Geometry: final body of the model. Coordinates: model frame, mm. A direction names the side the tool comes from. Give positions to 0.01 mm unless a question says otherwise; leave off trailing zeros. Loops run counter-clockwise (first coordinate to the right, second up) from the corner with the lowest first, then second, coordinate; pieces in that order, holes last. Notation, with made-up numbers: M -4.75,-9.75 L 12.25,-9.75 A13 ccw 12.25,7.25 Z; hole C 2.5,36.25 d3. An arc over 180 degrees is marked long. Put each result on its own line as item: value.
```python
from build123d import *

# Parameters (mm, degrees)
SKETCH2_W           = 42
SKETCH2_H           = 13.8
BOSS_EXTRUDE1_DEPTH = 2
SKETCH3_W           = 2
SKETCH3_H           = 13.8
BOSS_EXTRUDE2_DEPTH = 10
BOSS_EXTRUDE3_DEPTH = 2
SKETCH5_R           = 2.5
CUT_EXTRUDE1_DEPTH  = 2
SKETCH6_R           = 1.25
CUT_EXTRUDE2_DEPTH  = 2


with BuildPart() as part:
    # Sketch2 → Boss-Extrude1 (new body)
    with BuildSketch(Plane(origin=(0, 0, 0), x_dir=(1, 0, 0), z_dir=(0, 1, 0))):
        Rectangle(SKETCH2_W, SKETCH2_H)
    extrude(amount=BOSS_EXTRUDE1_DEPTH)

    # Sketch3 → Boss-Extrude2 (add)
    with BuildSketch(Plane.XZ):
        with Locations((-20, 0)):
            Rectangle(SKETCH3_W, SKETCH3_H)
        with Locations((20, 0)):
            Rectangle(SKETCH3_W, SKETCH3_H)
    extrude(amount=BOSS_EXTRUDE2_DEPTH)

    # Sketch4 → Boss-Extrude3 (add)
    with BuildSketch(Plane.XY.offset(6.9)):
        Polygon((-19, 0), (19, 0), (19, -10), (14, -5), (-14, -5), (-19, -10), align=None)
    boss_extrude3 = extrude(amount=-BOSS_EXTRUDE3_DEPTH)

    # Mirror1: Boss-Extrude3 across plane
    add(boss_extrude3.mirror(Plane.XY))

    # Sketch5 → Cut-Extrude1 (cut)
    with BuildSketch(Plane.XZ):
        with Locations((-8.319906625, 0)):
            Circle(SKETCH5_R)
        with Locations((6.680093375, 0)):
            Circle(SKETCH5_R)
    extrude(amount=-CUT_EXTRUDE1_DEPTH, mode=Mode.SUBTRACT)

    # Sketch6 → Cut-Extrude2 (cut)
    with BuildSketch(Plane(origin=(-19, 0, 0), x_dir=(0, 0, -1), z_dir=(1, 0, 0))):
        with Locations((-2.5, -3)):
            Circle(SKETCH6_R)
        with Locations((2.5, -3)):
            Circle(SKETCH6_R)
    cut_extrude2 = extrude(amount=-CUT_EXTRUDE2_DEPTH, mode=Mode.SUBTRACT)

    # Mirror2: Cut-Extrude2 across plane
    add(cut_extrude2.mirror(Plane(origin=(0, 0, 0), x_dir=(0, 0, 1), z_dir=(1, 0, 0))), mode=Mode.SUBTRACT)


solid = part.part
```
Item 1: Pin query (flat end, axial travel): pin 1 Ø1.5 at (x, z) = (-6.5, 3.5) entering from -Y; pin 2 Ø2 at (x, z) = (7, -6) entering from -Y. Return the tip coordinate at first contact, or that it passes through.
Output values:
pin 1: y = 0
pin 2: y = -5
Item 2: Section D-D on y = -5.75. Output: boundary loops of the cut face in (x, z).
Output values:
outline: M -21,-6.9 L -14.75,-6.9 L -14.75,-4.9 L -19,-4.9 L -19,4.9 L -14.75,4.9 L -14.75,6.9 L -21,6.9 Z; M 14.75,-6.9 L 21,-6.9 L 21,6.9 L 14.75,6.9 L 14.75,4.9 L 19,4.9 L 19,-4.9 L 14.75,-4.9 Z
Item 3: Section B-B on x = -4.5. Output: boundary loops of the cut face in (y, z).
Output values:
outline: M -5,-6.9 L 2,-6.9 L 2,6.9 L -5,6.9 L -5,4.9 L 0,4.9 L 0,-4.9 L -5,-4.9 Z
Item 4: Mould query, pull axis X, two halves, no side actions, for faces 1 (the flat face through (-21, -4, 0)), 2 (the flat face through (0, -5, 6)), 3 (the cylindrical face through (19.99, -2.62, -3.69)). Classes: pulls with the +X half, pulls with the -X half, needs draft (parallel to the pull), parting line crosses it, or undercut.
Output values:
face 1: pulls with the -X half
face 2: undercut
face 3: needs draft
Item 5: Line query: probe 1 along Z at (x, y) = (16, -4.5); probe 2 along Y at (x, z) = (-19.9, 2.5); probe 3 along X at (y, z) = (-9, 0). Output: solid intervals per line, ascending. Write a range as [from, to].
Output values:
probe 1: [-6.9, -4.9], [4.9, 6.9]
probe 2: [-10, -4.25], [-1.75, 2]
probe 3: [-21, -19], [19, 21]
Item 6: Set-up query: faces 4 (the flat face through (-19, -5, 0)), 5 (the cylindrical face through (-5.935, 0.986, 0.751)), 6 (the flat face through (-16, -7, 6)). Return all of +Z, -Z, +X, -X, +Y, -Y with unobstructed straight access to the full face (end or side cutting, diameter ignored); none if empty.
Output values:
face 4: -Y
face 5: +Y, -Y
face 6: +Z, -Z, -Y
Item 7: Section C-C on y = -3. Output: boundary loops of the cut face in (x, z).
Output values:
outline: M -21,-6.9 L 21,-6.9 L 21,-3.75 L 19,-3.75 L 19,-4.9 L -19,-4.9 L -19,-3.75 L -21,-3.75 Z; M -21,-1.25 L -19,-1.25 L -19,1.25 L -21,1.25 Z; M -21,3.75 L -19,3.75 L -19,4.9 L 19,4.9 L 19,3.75 L 21,3.75 L 21,6.9 L -21,6.9 Z; M 19,-1.25 L 21,-1.25 L 21,1.25 L 19,1.25 Z
Item 8: Section A-A on z = 0. Output: boundary loops of the cut face in (x, y), then the cut area to 3 significant figures.
Output values:
outline: M -21,-10 L -19,-10 L -19,0 L -10.82,0 L -10.82,2 L -21,2 Z; M -5.82,0 L 4.18,0 L 4.18,2 L -5.82,2 Z; M 9.18,0 L 19,0 L 19,-10 L 21,-10 L 21,2 L 9.18,2 Z
area: 104 mm²
